Source: CAD feature listing. Evaluate the final solid. Frame: model axes, mm. Give positions to 0.01 mm unless a question says otherwise; leave off trailing zeros. Loops run counter-clockwise (first coordinate to the right, second up) from the corner with the lowest first, then second, coordinate; pieces in that order, holes last. Notation, with made-up numbers: (38.5, 62) - (77.5, 62) arc R23 cw to (77.5, 86) - close; hole circle Ø1 at (59.5, -34). An arc over 180 degrees is marked (long way). Put each result on its own line as item: value.
```python
from build123d import *

# Parameters (mm, degrees)
F0_R     = 19.05
F0_R_2   = 3.175
F1_DEPTH = 30.48
F3_SIZE  = 1.27


with BuildPart() as f1:
    # F0 (on Right) → F1 (new body)
    with BuildSketch(Plane.YZ):
        Circle(F0_R)
        Circle(F0_R_2, mode=Mode.SUBTRACT)
    extrude(amount=F1_DEPTH)

    # F2: F1 across face


with BuildPart() as f1_1:
    add(f1.part)
    add(f1.part.mirror(Plane(origin=(0, 0, 0), x_dir=(0, 1, 0), z_dir=(-1, 0, 0))))

    # F3
    f3_edges = [f1_1.edges().sort_by_distance(p)[0] for p in [
        (30.48, -3.175, 0),
        (-30.48, -3.175, 0),
    ]]
    chamfer(f3_edges, length=F3_SIZE)


solid = f1_1.part
```
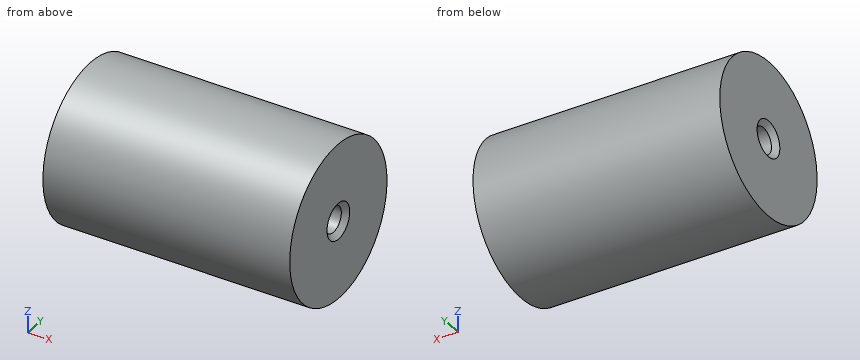
1) Material intervals for line 1 along Z through (x, y) = (-4, 0) (3 decimals); line 2 along Y through (x, z) = (4, 1); line 3 along Z through (x, y) = (-7.5, -17), sorted ascending. Write a range as [from, to].
Check result:
line 1: [-19.05, -3.175], [3.175, 19.05]
line 2: [-19.02, -3.01], [3.01, 19.02]
line 3: [-8.6, 8.6]
2) Section query C-C, the plane x = 3. Output: boundary loops of the cut face in (y, z) (3 decimals), plus the area to 3 significant figures.
Check result:
outline: circle Ø38.1 at (0, 0); hole circle Ø6.35 at (0, 0)
area: 1,110 mm²
3) Section query D-D, the plane z = -15.5. Output: boundary loops of the cut face in (x, y), plus the area to 3 significant figures.
Check result:
outline: (-30.48, -11.07) - (30.48, -11.07) - (30.48, 11.07) - (-30.48, 11.07) - close
area: 1,350 mm²
4) Section query A-A, the plane y = 0. Output: boundary loops of the cut face in (x, z) (3 decimals), plus the area to 3 significant figures.
Check result:
outline: (-30.48, -19.05) - (30.48, -19.05) - (30.48, -4.445) - (29.21, -3.175) - (-29.21, -3.175) - (-30.48, -4.445) - close; (-30.48, 4.445) - (-29.21, 3.175) - (29.21, 3.175) - (30.48, 4.445) - (30.48, 19.05) - (-30.48, 19.05) - close
area: 1,930 mm²
5) Pin query (flat end, axial travel): P1, Ø1.5, axis at y = -1, z = 2.5, coming from the -X side; P2, Ø1, axis at x = -20.5, y = 13.5, coming from the -Z side; P3, Ø8, axis at x = 21, z = -11.5, coming from the +Y side. Return the tip coordinate at first contact, or that it passes through.
Check result:
P1: x = -29.48
P2: z = -13.92
P3: y = 17.51
